Verification items for the finished model (mm, model axes). Face numbers are marked on the shaded views. Round coordinates to 2 decimals unless told otherwise and drop trailing zeros. Use a Markdown table: item, result. Add a question column.
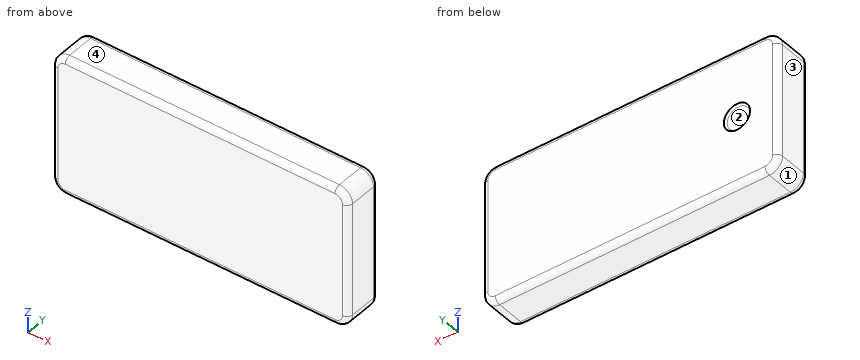
from build123d import *

# Parameters (mm, degrees)
BOSS_EXTRUDE1_DEPTH = 20.5
FILLET1_R           = 3
SKETCH2_R           = 7
CUT_EXTRUDE1_DEPTH  = 1
FILLET2_R           = 1


with BuildPart() as part:
    # Sketch1 → Boss-Extrude1 (new body)
    with BuildSketch(Plane(origin=(0, 0, 0), x_dir=(1, 0, 0), z_dir=(0, 1, 0))):
        with BuildLine():
            Line((7, 0), (151, 0))
            ThreePointArc((151, 0), (155.949747468, 2.050252532), (158, 7))
            Line((158, 7), (158, 67))
            ThreePointArc((158, 67), (155.949747468, 71.949747468), (151, 74))
            Line((151, 74), (7, 74))
            ThreePointArc((7, 74), (2.050252532, 71.949747468), (0, 67))
            Line((0, 67), (0, 7))
            ThreePointArc((0, 7), (2.050252532, 2.050252532), (7, 0))
        make_face()
    extrude(amount=BOSS_EXTRUDE1_DEPTH)

    # Fillet1
    fillet1_edges = [part.edges().sort_by_distance(p)[0] for p in [
        (0, 0, -37),
        (2.050252532, 0, -71.949747468),
        (79, 0, -74),
        (155.949747468, 0, -71.949747468),
        (2.050252532, 20.5, -71.949747468),
        (0, 20.5, -37),
        (2.050252532, 20.5, -2.050252532),
        (79, 20.5, 0),
        (155.949747468, 20.5, -2.050252532),
        (158, 20.5, -37),
        (155.949747468, 20.5, -71.949747468),
        (158, 0, -37),
        (79, 20.5, -74),
        (155.949747468, 0, -2.050252532),
        (79, 0, 0),
        (2.050252532, 0, -2.050252532),
    ]]
    fillet(fillet1_edges, radius=FILLET1_R)

    # Sketch2 → Cut-Extrude1 (cut)
    with BuildSketch(Plane(origin=(0, 20.5, 0), x_dir=(1, 0, 0), z_dir=(0, 1, 0))):
        with Locations(Location((22, 37, 0), (0, 0, 270))):
            Circle(SKETCH2_R)
    extrude(amount=-CUT_EXTRUDE1_DEPTH, mode=Mode.SUBTRACT)

    # Fillet2
    fillet2_edges = [part.edges().sort_by_distance(p)[0] for p in [
        (22, 19.5, -44),
    ]]
    fillet(fillet2_edges, radius=FILLET2_R - 0.0001)  # a hair under: the kernel refuses the full size


solid = part.part
1. Depth check by flat-ended pin: pin 1 Ø6 at (x, z) = (24, -40) entering from +Y. Enter the tip coordinate at first touch or a pass-through.
2. Release check for a two-part mould opening along Z. For the marked faces 1, 2, 3 and 4 record: +Z half, -Z half, draft (parallel to the pull), parting line (faces both ways), or undercut.
3. Scan lines: line 1 along X through (y, z) = (18.5, -12); line 2 along X through (y, z) = (2.25, -24.5); line 3 along Z through (x, y) = (44.5, 19.5). Record each from-to range of solid material in increasing order. Write a range as from..to.
Answer:
| question | item | result |
|---|---|---|
| 1 | pin 1 | stops at y = 19.7 |
| 2 | face 1 | -Z half |
| 2 | face 2 | undercut |
| 2 | face 3 | draft |
| 2 | face 4 | +Z half |
| 3 | line 1 | x = 0.17..157.83 |
| 3 | line 2 | x = 0.1..157.9 |
| 3 | line 3 | z = -73.24..-0.76 |
